Geometry: final body of the model. Coordinates: model frame, mm. Face numbers are marked on the shaded views. A direction names the side the tool comes from. Round coordinates to 2 decimals unless told otherwise and drop trailing zeros. Write each loop counter-clockwise with the first axis right and the second up, starting at its lowest first coordinate (ties: lowest second). Pieces come first, ordered by that corner, then holes. Notation, with made-up numbers: (12.25, 4) -> (56.25, 4) arc R17 ccw to (56.25, 9) -> close; hole circle Ø1 at (-23, 12). An arc over 180 degrees is marked (long way). Use one line per item in the form item = value. Start each with the question number.
1. Cut plane D-D, the plane z = 0. Return the cut outline in (x, y) (3 decimals).
2. Pin query (flat end, axial travel): pin 1 Ø7 at (x, y) = (-0.5, -1) entering from +Z; pin 2 Ø1 at (y, z) = (-1, -6.5) entering from -X; pin 3 Ø3.5 at (x, y) = (-2, 1) entering from -Z. Return the tip coordinate at first contact, or that it passes through.
3. Cut plane A-A, the plane y = 0. State how many separate pieces and enclosed holes the cut face has, plus the area to 3 significant figures.
4. Reachability of the marked faces 5, 6 and 7 from +Z, -Z, +X, -X, +Y, -Y: full face, straight path, thin tool, end or side. Return the list, or none.
5. Cut plane B-B, the plane z = 12.75. Return the cut outline in (x, y) (3 decimals), plus the area to 3 significant figures.
6. Line query: L1, parallel to Y at x = 0, z = 12.05 (3 decimals); L2, parallel to Z at x = 0, y = -8.7; L3, parallel to Z at x = 6, y = 1. Output: solid intervals per line, ascending.
7. Draft query along Z for the marked faces 1, 2, 3 and 4. Return one class per face: pulls with the +Z half, pulls with the -Z half, needs draft (parallel to the pull), parting line crosses it, or undercut.
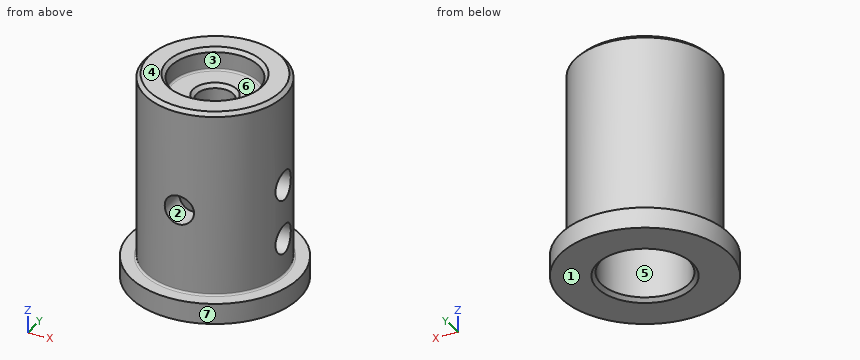
```python
from build123d import *

# Parameters (mm, degrees)
SKETCH3_W          = 2.83
SKETCH3_H          = 2
CHAMFER1_SIZE      = 0.5
FILLET1_R          = 0.25
SKETCH4_R          = 2
CUT_EXTRUDE2_DEPTH = 22.616920456
SKETCH5_R          = 2
CUT_EXTRUDE3_DEPTH = 22.616920456


with BuildPart() as part:
    # Sketch1 → Revolve1 (revolve)
    with BuildSketch(Plane(origin=(0, 0, 0), x_dir=(0, 0, -1), z_dir=(1, 0, 0)), mode=Mode.PRIVATE) as revolve1_sk:
        Polygon((-14.2, 6), (-14.2, 9.525), (14.2, 9.525), (14.2, 6), (-6.8, 6), (-6.8, 2.5), (-11.2, 2.5), (-11.2, 6), align=None)
    revolve(revolve1_sk.sketch.rotate(Axis((0, 0, 14.2), (0, 0, -1)), 90), axis=Axis((0, 0, 14.2), (0, 0, -1)))

    # Sketch3 → Revolve2 (revolve)
    with BuildSketch(Plane(origin=(0, 0, 0), x_dir=(0, 0, -1), z_dir=(1, 0, 0)), mode=Mode.PRIVATE) as revolve2_sk:
        with Locations((12.785, 10.525)):
            Rectangle(SKETCH3_W, SKETCH3_H)
    revolve(revolve2_sk.sketch.rotate(Axis((0, 0, 0), (0, 0, -1)), 90), axis=Axis((0, 0, 0), (0, 0, -1)))

    # Chamfer1
    chamfer1_edges = [part.edges().sort_by_distance(p)[0] for p in [
        (-2.5, 0, 11.2),
        (-6, 0, -14.2),
        (-9.525, 0, 14.2),
        (-6, 0, 14.2),
    ]]
    chamfer(chamfer1_edges, length=CHAMFER1_SIZE)

    # Fillet1
    fillet1_edges = [part.edges().sort_by_distance(p)[0] for p in [
        (-9.525, 0, -11.37),
        (-6, 0, 11.2),
    ]]
    fillet(fillet1_edges, radius=FILLET1_R)

    # Sketch4 → Cut-Extrude2 (cut, through all)
    with BuildSketch(Plane(origin=(0, 0, 0), x_dir=(0, 0, -1), z_dir=(1, 0, 0))):
        with Locations((6.37, 0)):
            Circle(SKETCH4_R)
        with Locations((-1.13, 0)):
            Circle(SKETCH4_R)
    extrude(amount=CUT_EXTRUDE2_DEPTH, mode=Mode.SUBTRACT)

    # Sketch5 → Cut-Extrude3 (cut, through all)
    with BuildSketch(Plane(origin=(0, 0, 0), x_dir=(1, 0, 0), z_dir=(0, 1, 0))):
        with Locations(Location((0, 0, 0), (0, 0, 270))):
            Circle(SKETCH5_R)
    extrude(amount=-CUT_EXTRUDE3_DEPTH, mode=Mode.SUBTRACT)


solid = part.part
```
Outcome:
q1.outline = (-2, -9.313) -> (-2, -5.657) arc R6 cw (long way) to (5.769, 1.65) -> (9.381, 1.65) arc R9.525 ccw (long way) to start; (2, -9.313) arc R9.525 ccw to (9.381, -1.65) -> (5.769, -1.65) arc R6 cw to (2, -5.657) -> close
q2.pin_1 = 11.2
q2.pin_2 = -9.51
q2.pin_3 = 6.8
q3.separate_pieces = 4
q3.enclosed_holes = 0
q3.area = 213 mm^2
q4.face_5 = -Z
q4.face_6 = +Z
q4.face_7 = +Z, -Z
q5.outline = circle Ø19.05 at (0, 0); hole circle Ø12 at (0, 0)
q5.area = 172 mm^2
q6.L1 = -9.525 to -6, 6 to 9.525
q6.L2 = -14.2 to -2, 2 to 14.2
q6.L3 = -13.78 to -8.1, -4.64 to -0.6, 2.86 to 13.78
q7.face_1 = pulls with the -Z half
q7.face_2 = undercut
q7.face_3 = needs draft
q7.face_4 = pulls with the +Z half
